from build123d import *

# Parameters (mm, degrees)
F0_W      = 9.6
F0_H      = 19
F1_DEPTH  = 8
F2_W      = 4
F2_H      = 19
F2_W_2    = 9.6
F3_DEPTH  = 5
F4_W      = 4
F4_H      = 19
F5_DEPTH  = 10
F6_R      = 2
F7_DEPTH  = 4
F6_R_2    = 3.1
F8_DEPTH  = 1.5
F9_W      = 17.6
F9_H      = 7.5
F10_DEPTH = 25
F11_W     = 10
F11_H     = 7.5
F12_DEPTH = 70
F14_DEPTH = 25
F15_DEPTH = 40
F16_R     = 1.5
F17_DEPTH = 25
F18_DEPTH = 25
F20_DEPTH = 25
F21_R     = 4.99999


# Not quite as in the source:
# - a fillet or chamfer is up to 0.001 mm smaller than in the source, because OpenCascade refuses the exact size


with BuildPart() as f1:
    # F0 (on Front) → F1 (new body)
    with BuildSketch(Plane.XZ):
        Rectangle(F0_W, F0_H)
    extrude(amount=F1_DEPTH)

    # F2 (on face) → F3 (join)
    with BuildSketch(Plane(origin=(0, 0, 0), x_dir=(-1, 0, 0), z_dir=(0, 1, 0))):
        with Locations((6.8, 0)):
            Rectangle(F2_W, F2_H)
        Rectangle(F2_W_2, F2_H)
        with Locations((10.8, 0)):
            Rectangle(F2_W, F2_H)
    extrude(amount=F3_DEPTH)

    # F4 (on face) → F5 (join)
    with BuildSketch(Plane.XZ):
        with Locations((-10.8, 0)):
            Rectangle(F4_W, F4_H)
    extrude(amount=F5_DEPTH)

    # F6 (on face) → F7 (cut, through all)
    with BuildSketch(Plane(origin=(-12.8, 0, 0), x_dir=(0, -1, 0), z_dir=(-1, 0, 0))):
        with Locations((3, 0)):
            Circle(F6_R)
    extrude(amount=-F7_DEPTH, mode=Mode.SUBTRACT)

    # F6 (on face) → F8 (cut)
    with BuildSketch(Plane(origin=(-12.8, 0, 0), x_dir=(0, -1, 0), z_dir=(-1, 0, 0))):
        with Locations((3, 0)):
            Circle(F6_R_2)
        with Locations((3, 0)):
            Circle(F6_R, mode=Mode.SUBTRACT)
    extrude(amount=-F8_DEPTH, mode=Mode.SUBTRACT)

    # F9 (on face) → F10 (join)
    with BuildSketch(Plane(origin=(0, 5, 0), x_dir=(-1, 0, 0), z_dir=(0, 1, 0))):
        with Locations((4, -5.75)):
            Rectangle(F9_W, F9_H)
    extrude(amount=F10_DEPTH)

    # F11 (on face) → F12 (join)
    with BuildSketch(Plane.YZ.offset(4.8)):
        with Locations((25, -5.75)):
            Rectangle(F11_W, F11_H)
    extrude(amount=F12_DEPTH)

    # F13 (on face) → F14 (cut)
    with BuildSketch(Plane.XY.offset(-2)):
        Polygon((74.8, 30), (64.8, 20), (74.8, 20), align=None)
    extrude(amount=-F14_DEPTH, mode=Mode.SUBTRACT)

    # F15 (add): a face of the model
    f15_faces = [f1.faces().sort_by_distance(p)[0] for p in [
        (69.8, 25, -5.75),
    ]]
    extrude(f15_faces, amount=F15_DEPTH)

    # F16 (on face) → F17 (cut)
    with BuildSketch(Plane.XY.offset(-2)):
        with Locations((96.0132034356, 1.7157287525)):
            Circle(F16_R)
    extrude(amount=-F17_DEPTH, mode=Mode.SUBTRACT)

    # F18 (add): a face of the model
    f18_faces = [f1.faces().sort_by_distance(p)[0] for p in [
        (-4, 5, 3.75),
    ]]
    extrude(f18_faces, amount=F18_DEPTH)

    # F19 (on face) → F20 (cut)
    with BuildSketch(Plane.XY.offset(-2)):
        Polygon((93.0842712475, -8.2842712475), (96.0132034356, -5.3553390593), (70.6578643763, 20), (64.8, 20), align=None)
    extrude(amount=-F20_DEPTH, mode=Mode.SUBTRACT)

    # F21 (radius 5 in the source; OpenCascade refuses exactly that, so slightly less here)
    f21_edges = [f1.edges().sort_by_distance(p)[0] for p in [
        (96.013203, -5.355339, -5.75),
        (103.084271, 1.715729, -5.75),
    ]]
    fillet(f21_edges, radius=F21_R)


solid = f1.part
Input: part model. Units: mm. Frame: model coordinates. A direction names the side the tool comes from. Coordinates: 2 decimals unless noted, no trailing zeros. Loops run counter-clockwise (first coordinate to the right, second up) from the corner with the lowest first, then second, coordinate; pieces in that order, holes last.
(1) Section B-B on z = 5.5. Return the cut outline in (x, y), then the cut area to 3 significant figures.
(2) Material intervals for probe 1 along X at (y, z) = (-4.5, 8.5); probe 2 along Z at (x, y) = (-12, -3); probe 3 along X at (y, z) = (12, 2.25), sorted ascending.
(3) First-contact query: pin 1 Ø10 at (y, z) = (-6, -5.5) entering from +X; pin 2 Ø5.5 at (y, z) = (11.5, -4.5) entering from +X; pin 3 Ø8 at (x, z) = (43, -6.5) entering from -Y. Flat tips, straight axial feed; report the tip coordinate or a pass-through.
(4) Pull-direction query (Z, two-part tool) for faces 4 (the face through (-12.8, 10, 0)), 5 (the face through (-11.3, -5, -1)), 6 (the face through (-10, -3, -2)), 7 (the face through (34, 21, -9.5)); classes: released by +Z, released by -Z, zero draft, split by the parting line, or undercut.
(5) Section A-A on z = 0. Return the cut outline in (x, y).
(6) Section C-C on y = 10. Return the cut outline in (x, z), then the cut area to 3 significant figures.
(7) Set-up query: faces 1 (the face through (4.8, 11, 0)), 2 (the face through (81.72, 8.94, -5.7)), 3 (the face through (-12.061, -2.328, -3.026)). Return all of +Z, -Z, +X, -X, +Y, -Y with unobstructed straight access to the full face (end or side cutting, diameter ignored); none if empty.
Data:
1. outline: (-12.8, -10) - (-8.8, -10) - (-8.8, 0) - (-4.8, 0) - (-4.8, -8) - (4.8, -8) - (4.8, 30) - (-12.8, 30) - close
1. area: 645 mm2
2. probe 1: x = -12.8 to -8.8, -4.8 to 4.8
2. probe 2: z = -9.5 to -3.1, 3.1 to 9.5
2. probe 3: x = -12.8 to 4.8
3. pin 1: stops at x = 100.21
3. pin 2: stops at x = 96.05
3. pin 3: stops at y = 20
4. face 4: zero draft
4. face 5: undercut
4. face 6: undercut
4. face 7: released by -Z
5. outline: (-12.8, -10) - (-8.8, -10) - (-8.8, -5) - (-11.3, -5) - (-11.3, -6.1) - (-12.8, -6.1) - close; (-12.8, 0.1) - (-11.3, 0.1) - (-11.3, -1) - (-8.8, -1) - (-8.8, 0) - (-4.8, 0) - (-4.8, -8) - (4.8, -8) - (4.8, 30) - (-12.8, 30) - close
6. outline: (-12.8, -9.5) - (4.8, -9.5) - (4.8, 9.5) - (-12.8, 9.5) - close; (80.66, -9.5) - (94.8, -9.5) - (94.8, -2) - (80.66, -2) - close
6. area: 440 mm2
7. face 1: +Z, -Y
7. face 2: +Z, -Z, -Y
7. face 3: -X
